Check sheet for the modelled part. Datum: model origin and axes. Units: mm. A direction names the side the tool comes from. Give positions to 0.01 mm unless a question says otherwise; leave off trailing zeros. Order: outer loops, then holes, each group sorted by start corner. A loop starts at its lowest first (then second) coordinate and runs counter-clockwise, first axis right, second up.
from build123d import *

# Parameters (mm, degrees)
F0_W     = 60
F0_H     = 15
F1_DEPTH = 30
F3_DEPTH = 60.001
F4_W     = 20
F4_H     = 12
F5_DEPTH = 30.001
F6_R     = 1.65
F7_DEPTH = 15.001
F8_R     = 2
F9_DEPTH = 15.001


with BuildPart() as f1:
    # F0 (on Front) → F1 (new body)
    with BuildSketch(Plane.XZ):
        Rectangle(F0_W, F0_H)
    extrude(amount=F1_DEPTH)

    # F2 (on face) → F3 (cut, through all)
    with BuildSketch(Plane(origin=(-30, 0, 0), x_dir=(0, -1, 0), z_dir=(-1, 0, 0))):
        Polygon((8.1, 3.25), (0, 3.25), (0, -3.25), (2, -3.25), (2, -2.25), (5.6, -2.25), (5.6, -3.25), (8.1, -3.25), (8.1, -0.5), (27, -0.5), (27, 0.5), (8.1, 0.5), align=None)
    extrude(amount=-F3_DEPTH, mode=Mode.SUBTRACT)

    # F4 (on face) → F5 (cut, through all)
    with BuildSketch(Plane.XZ.offset(30)):
        with Locations((20, -1.5)):
            Rectangle(F4_W, F4_H)
    extrude(amount=-F5_DEPTH, mode=Mode.SUBTRACT)

    # F6 (on face) → F7 (cut, through all)
    with BuildSketch(Plane(origin=(0, 0, -7.5), x_dir=(1, 0, 0), z_dir=(0, 0, -1))):
        with Locations((5, 11.1)):
            Circle(F6_R)
        with Locations((-25, 11.1)):
            Circle(F6_R)
        with Locations((-10, 11.1)):
            Circle(F6_R)
    extrude(amount=-F7_DEPTH, mode=Mode.SUBTRACT)

    # F8 (on face) → F9 (cut, through all)
    with BuildSketch(Plane.XY.offset(7.5)):
        with Locations((22.77234, -23.078762)):
            Circle(F8_R)
    extrude(amount=-F9_DEPTH, mode=Mode.SUBTRACT)


solid = f1.part
1) Set-up check for faces 1 (the face through (-10, -7, -3.25)), 2 (the face through (10, -15, -2)), 3 (the face through (-10, -17, -0.5)): record each of +Z, -Z, +X, -X, +Y, -Y from which the full face is reachable in a straight line by a thin tool's end or side.
Recorded:
face 1: +X, -X
face 2: -Z, +X, +Y, -Y
face 3: +X, -X, +Y
2) Section check B-B, the plane z = -1.25. Record the cut outline in (x, y), then the cut area to 3 significant figures.
Recorded:
outline: (-30, -30) - (10, -30) - (10, -8.1) - (-30, -8.1) - close; hole circle Ø3.3 at (-25, -11.1); hole circle Ø3.3 at (-10, -11.1); hole circle Ø3.3 at (5, -11.1)
area: 850 mm2
3) Section check D-D, the plane y = -17.25. Record the cut outline in (x, z).
Recorded:
outline: (-30, -7.5) - (10, -7.5) - (10, -0.5) - (-30, -0.5) - close; (-30, 0.5) - (10, 0.5) - (10, 4.5) - (30, 4.5) - (30, 7.5) - (-30, 7.5) - close
4) Section check A-A, the plane y = -11.1. State how many separate pieces and enclosed holes the cut face has, then the cut area to 3 significant figures.
Recorded:
separate pieces: 8
enclosed holes: 0
area: 481 mm2
5) Depth check by flat-ended pin: pin 1 Ø4 at (x, y) = (-10, -11.1) entering from +Z; pin 2 Ø3 at (x, z) = (-13.5, -1.5) entering from +Y; pin 3 Ø0.8 at (x, z) = (-13.5, 2.5) entering from +Y; pin 4 Ø16 at (x, y) = (24, -18) entering from -Z. Enter the tip coordinate at first touch or a pass-through.
Recorded:
pin 1: stops at z = 7.5
pin 2: stops at y = -2
pin 3: stops at y = -8.1
pin 4: stops at z = 4.5
6) Material ranges on L1, parallel to Y at x = 5, z = -2.75; L2, parallel to X at y = -11.1, z = 5.75; L3, parallel to X at y = -11.1, z = -5.5, recorded low to high.
Recorded:
L1: y = -30 to -12.75, -9.45 to -8.1, -5.6 to -2
L2: x = -30 to -26.65, -23.35 to -11.65, -8.35 to 3.35, 6.65 to 30
L3: x = -30 to -26.65, -23.35 to -11.65, -8.35 to 3.35, 6.65 to 10
7) Draft check along Z on faces 4 (the face through (0, -15, 7.5)), 5 (the face through (-10, -8.1, -2)), 6 (the face through (-10, -15, -7.5)). Enter one of: +Z half, -Z half, draft (parallel to the pull), parting line (faces both ways), or undercut.
Recorded:
face 4: +Z half
face 5: undercut
face 6: -Z half
8) Section check C-C, the plane x = -10. Record the cut outline in (y, z), then the cut area to 3 significant figures.
Recorded:
outline: (-30, -7.5) - (-12.75, -7.5) - (-12.75, -0.5) - (-27, -0.5) - (-27, 0.5) - (-12.75, 0.5) - (-12.75, 7.5) - (-30, 7.5) - close; (-9.45, -7.5) - (0, -7.5) - (0, -3.25) - (-2, -3.25) - (-2, -2.25) - (-5.6, -2.25) - (-5.6, -3.25) - (-8.1, -3.25) - (-8.1, -0.5) - (-9.45, -0.5) - close; (-9.45, 0.5) - (-8.1, 0.5) - (-8.1, 3.25) - (0, 3.25) - (0, 7.5) - (-9.45, 7.5) - close
area: 336 mm2
